from build123d import *

# Parameters (mm, degrees)
SKETCH1_W                       = 150
SKETCH1_H                       = 36
BOSS_EXTRUDE1_DEPTH             = 2.4
SKETCH10_W                      = 75
SKETCH10_H                      = 9
CUT_EXTRUDE5_DEPTH              = 10
SKETCH2_R                       = 1.4
CUT_EXTRUDE1_DEPTH              = 155.278190293
CHAMFER6_SIZE                   = 9
SKETCH3_W                       = 5
SKETCH3_H                       = 50
BOSS_EXTRUDE2_DEPTH             = 30
BOSS_EXTRUDE2_DIRECTION_2_REACH = 156.278
SKETCH4_R                       = 3.15
CUT_EXTRUDE2_DEPTH              = 30
SKETCH8_W                       = 10
SKETCH8_H                       = 2
BOSS_EXTRUDE4_DEPTH             = 145
SKETCH9_W                       = 20
SKETCH9_H                       = 12.540874848
SKETCH9_H_2                     = 13.006860614
CUT_EXTRUDE4_DEPTH              = 161.934769394
CHAMFER5_SIZE                   = 6


with BuildPart() as part:
    # Sketch1 → Boss-Extrude1 (new body)
    with BuildSketch(Plane.XY):
        with Locations((75, 18)):
            Rectangle(SKETCH1_W, SKETCH1_H)
    extrude(amount=BOSS_EXTRUDE1_DEPTH)

    # Sketch10 → Cut-Extrude5 (cut)
    with BuildSketch(Plane.XY.offset(2.4)):
        with Locations((37.5, 31.5)):
            Rectangle(SKETCH10_W, SKETCH10_H)
    extrude(amount=-CUT_EXTRUDE5_DEPTH, mode=Mode.SUBTRACT)

    # Sketch2 → Cut-Extrude1 (cut, through all)
    with BuildSketch(Plane.XY.offset(2.4)):
        with Locations((40, 22.5)):
            Circle(SKETCH2_R)
        with Locations(Location((10, 22.5, 0), (0, 0, 180))):
            Circle(SKETCH2_R)
        with Locations(Location((106.5, 31.5, 0), (0, 0, 180))):
            Circle(SKETCH2_R)
        with Locations((136.5, 31.5)):
            Circle(SKETCH2_R)
        Polygon((131.5, 36), (126.5, 24), (116.5, 24), (111.5, 36), align=None)
        Polygon((35, 27), (30, 15), (20, 15), (15, 27), align=None)
    extrude(amount=-CUT_EXTRUDE1_DEPTH, mode=Mode.SUBTRACT)

    # Chamfer6
    chamfer6_edges = [part.edges().sort_by_distance(p)[0] for p in [
        (75, 27, 1.2),
    ]]
    chamfer(chamfer6_edges, length=CHAMFER6_SIZE - 0.0001)  # a hair under: the kernel refuses the full size

    # Sketch3 → Boss-Extrude2 (add)
    with BuildSketch(Plane(origin=(0, 0, 0), x_dir=(-1, 0, 0), z_dir=(0, 0, -1))):
        with Locations((-147.5, 11)):
            Rectangle(SKETCH3_W, SKETCH3_H)
    extrude(amount=BOSS_EXTRUDE2_DEPTH)

    # Boss-Extrude2 direction 2: up to this face of the body (flat: up to its plane)
    boss_extrude2_direction_2_end = Plane(part.part.faces().sort_by_distance((80.903875834, 15.309167909, 2.4))[0])
    # Sketch3 → Boss-Extrude2 direction 2 (add, up to the picked face)
    with BuildSketch(Plane(origin=(0, 0, 0), x_dir=(-1, 0, 0), z_dir=(0, 0, -1)), mode=Mode.PRIVATE) as boss_extrude2_direction_2_sk1:
        with Locations((-147.5, 11)):
            Rectangle(SKETCH3_W, SKETCH3_H)
    boss_extrude2_direction_2_tool1 = split(extrude(boss_extrude2_direction_2_sk1.sketch, amount=-BOSS_EXTRUDE2_DIRECTION_2_REACH, mode=Mode.PRIVATE), bisect_by=boss_extrude2_direction_2_end, keep=Keep.BOTH, mode=Mode.PRIVATE)
    add(boss_extrude2_direction_2_tool1.solids().sort_by(Axis((147.5, 11, 0), (0, 0, 1)))[0])

    # Sketch4 → Cut-Extrude2 (cut)
    with BuildSketch(Plane.ZY.offset(-145)):
        with Locations((-13.6, 27)):
            Circle(SKETCH4_R)
        with Locations((-13.6, -5)):
            Circle(SKETCH4_R)
    extrude(amount=-CUT_EXTRUDE2_DEPTH, mode=Mode.SUBTRACT)

    # Sketch8 → Boss-Extrude4 (add)
    with BuildSketch(Plane.ZY.offset(-145)):
        with Locations((-5, 11)):
            Rectangle(SKETCH8_W, SKETCH8_H)
    extrude(amount=BOSS_EXTRUDE4_DEPTH)

    # Sketch9 → Cut-Extrude4 (cut, through all)
    with BuildSketch(Plane(origin=(0, 36, 0), x_dir=(1, 0, 0), z_dir=(0, 1, 0))):
        with Locations((121.5, 6.270437424)):
            Rectangle(SKETCH9_W, SKETCH9_H)
        with Locations((25, 6.503430307)):
            Rectangle(SKETCH9_W, SKETCH9_H_2)
    extrude(amount=-CUT_EXTRUDE4_DEPTH, mode=Mode.SUBTRACT)

    # Chamfer5
    chamfer5_edges = [part.edges().sort_by_distance(p)[0] for p in [
        (0, 11, -10),
        (111.5, 11, -10),
        (131.5, 11, -10),
        (15, 11, -10),
        (35, 11, -10),
    ]]
    chamfer(chamfer5_edges, length=CHAMFER5_SIZE)


solid = part.part
The model under review builds one solid part; all positions refer to its coordinate system, in mm. A direction names the side the tool comes from. Round coordinates to 2 decimals unless told otherwise and drop trailing zeros. Loops run counter-clockwise (first coordinate to the right, second up) from the corner with the lowest first, then second, coordinate; pieces in that order, holes last. Notation, with made-up numbers: (2, 39) -> (44, 39) arc R33 cw to (44, 78) -> close; hole circle Ø10 at (59.5, 59). An arc over 180 degrees is marked (long way). Return JSON: item names as keys, results as strings.
(1) Add section B-B on y = -5. Write out the cut boundary in (x, z).
Solved:
{"outline": "(145, -30) -> (150, -30) -> (150, -16.75) -> (145, -16.75) -> close; (145, -10.45) -> (150, -10.45) -> (150, 2.4) -> (145, 2.4) -> close"}
(2) For faces 4 (the flat face through (32.535, 21.084, 1.217)), 5 (the flat face through (74, 12, -5)), 6 (the flat face through (134.5, 11, -7)), 7 (the flat face through (74, 10, -5)), list the 3-axis set-ups (+Z, -Z, +X, -X, +Y, -Y) from which the entire face can be reached by the end or side of a thin tool; tool diameter is ignored.
Solved:
{"face 4": "+Z, -Z, +Y", "face 5": "-Z, -X, +Y", "face 6": "-Z, +Y, -Y", "face 7": "-Z, -X, -Y"}
(3) Add section C-C on y = 31.5. Write out the cut boundary in (x, z) (3 decimals).
Solved:
{"outline": "(70.5, 0) -> (105.1, 0) -> (105.1, 2.4) -> (70.5, 2.4) -> close; (107.9, 0) -> (113.375, 0) -> (113.375, 2.4) -> (107.9, 2.4) -> close; (129.625, 0) -> (135.1, 0) -> (135.1, 2.4) -> (129.625, 2.4) -> close; (137.9, 0) -> (145, 0) -> (145, -30) -> (150, -30) -> (150, 2.4) -> (137.9, 2.4) -> close"}
(4) The part is to be moulded in two halves that separate along X. For faces 1 (the flat face through (150, 11, -14)), 2 (the cylindrical face through (135.1, 31.56, 1.22)), 3 (the flat face through (146, 36, -10)), say which applies: released by +X, released by -X, zero draft, split by the parting line, or undercut.
Solved:
{"face 1": "released by +X", "face 2": "undercut", "face 3": "zero draft"}
(5) Add section A-A on z = -13.6. Write out the cut boundary in (x, y).
Solved:
{"outline": "(145, -14) -> (150, -14) -> (150, -8.15) -> (145, -8.15) -> close; (145, -1.85) -> (150, -1.85) -> (150, 23.85) -> (145, 23.85) -> close; (145, 30.15) -> (150, 30.15) -> (150, 36) -> (145, 36) -> close"}
(6) For pin 1 (11 mm diameter, centred on x = 7.5, z = -3.5, fed in from +Y); pin 2 (1 mm diameter, centred on x = 7, y = 11, fed in from -Z); pin 3 (2.5 mm diameter, centred on x = 77, z = 1, fed in from -Y), all flat-tipped, find the tip position at first contact; note any pin that passes through.
Solved:
{"pin 1": "y = 27", "pin 2": "z = -10", "pin 3": "y = 0"}
(7) Add section D-D on z = -5.5. Write out the cut boundary in (x, y), plus the area to 3 significant figures.
Solved:
{"outline": "(1.5, 10) -> (13.5, 10) -> (13.5, 12) -> (1.5, 12) -> close; (36.5, 10) -> (110, 10) -> (110, 12) -> (36.5, 12) -> close; (133, 10) -> (145, 10) -> (145, -14) -> (150, -14) -> (150, 36) -> (145, 36) -> (145, 12) -> (133, 12) -> close", "area": "445 mm2"}
(8) For line 1 (Y direction, x = 147.2, z = -13.6); line 2 (Y direction, x = 40, z = 0.6); line 3 (X direction, y = 18, z = -16.5), list the stretches that pass through material, from the lowest coordinate up.
Solved:
{"line 1": "-14 to -8.15, -1.85 to 23.85, 30.15 to 36", "line 2": "0 to 21.1, 23.9 to 27", "line 3": "145 to 150"}
